Build history of the part. All positions in model axes, mm. A direction names the side the tool comes from. Round coordinates to 2 decimals unless told otherwise and drop trailing zeros. Order: outer loops, then holes, each group sorted by start corner. A loop starts at its lowest first (then second) coordinate and runs counter-clockwise, first axis right, second up. Notation, with made-up numbers: (74.5, 54.5) -> (131.5, 54.5) arc R25 cw to (131.5, 75.5) -> close; hole circle Ø6 at (69.25, -17.75). An arc over 180 degrees is marked (long way). Use a Markdown table: item, result. Add a question column.
Item 1: Two-plate mould, pull along Y, no slides. Class faces 1 (the face through (6.794, -4.514, 1.62)), 2 (the face through (0, -6, -8)), 3 (the face through (0.48, -0.25, 14.84)): released by +Y, released by -Y, zero draft, split by the parting line, or undercut.
Item 2: Slice it at A-A, the plane z = 11. Give the cut face in (x, y), plus the area to 3 significant figures.
Item 3: Pin check, flat tips, straight feed: pin 1 (4 mm diameter, centred on x = 3, z = 3.5, fed in from +Y); pin 2 (2 mm diameter, centred on x = 6, z = 7, fed in from -Y); pin 3 (8 mm diameter, centred on y = -1.5, z = -10, fed in from +X). Stop position of each tip, or through.
Item 4: Probe L1, parallel to Z at x = -6, y = -3.25; L2, parallel to Z at x = -2.75, y = -4.75 (3 decimals); L3, parallel to Y at x = 6.5, z = 13.5. List the from-to ranges inside material, lowest first.
Item 5: Slice it at B-B, the plane z = -12. Give the cut face in (x, y).
Item 6: 3-axis set-ups, long thin cutter, end or side, ignore diameter. For faces 4 (the face through (0, -10, 5)), 5 (the face through (-1.6, -5, 0.9)), 6 (the face through (-6.2, -0.1, 1.5)): which of +Z, -Z, +X, -X, +Y, -Y reach the whole face in a straight line?
from build123d import *

# Parameters (mm, degrees)
CUT_EXTRUDE4_DEPTH = 23.891046285
FILLET1_R          = 0.4
FILLET2_R          = 0.4
FILLET3_R          = 0.3


with BuildPart() as part:
    # Sketch3 → Revolve2 (revolve)
    with BuildSketch(Plane(origin=(0, 0, 0), x_dir=(0, 0, -1), z_dir=(1, 0, 0))):
        Polygon((-16.5, 0), (-16.5, 8.004748036), (-7.5, 10), (-1.5, 10), (-1.5, 6), (16.5, 6), (16.5, 0), align=None)
    revolve(axis=Axis((0, 0, -16.5), (0, 0, 1)))

    # Sketch14 → Cut-Extrude4 (cut, through all)
    with BuildSketch(Plane(origin=(0, 0, 1.5), x_dir=(-1, 0, 0), z_dir=(0, 0, -1))):
        Polygon((-9.531762002, 0), (-4.326626661, -9.01555887), (0.878508679, -18.03111774), (-12.531762002, -18.03111774), (-12.531762002, 18.03111774), (0.878508679, 18.03111774), (-4.326626661, 9.01555887), align=None)
    cut_extrude4 = extrude(amount=-CUT_EXTRUDE4_DEPTH, mode=Mode.SUBTRACT)

    # Mirror1: Cut-Extrude4 across plane
    add(cut_extrude4.mirror(Plane(origin=(0, 0, 0), x_dir=(0, 0, 1), z_dir=(1, 0, 0))), mode=Mode.SUBTRACT)

    # Sketch16 → Cut-Revolve1 (revolve, cut)
    with BuildSketch(Plane(origin=(0, 0, 0), x_dir=(0, 0, -1), z_dir=(1, 0, 0)), mode=Mode.PRIVATE) as cut_revolve1_sk:
        with BuildLine():
            Line((-1.5, 6), (-1.716506351, 5.625))
            ThreePointArc((-1.716506351, 5.625), (-1.716506351, 5.375), (-1.5, 5.25))
            Line((-1.5, 5.25), (-0.225098536, 5.25))
            ThreePointArc((-0.225098536, 5.25), (0.035373731, 5.27278837), (0.287931679, 5.340461069))
            Line((0.287931679, 5.340461069), (2.1, 6))
            Line((2.1, 6), (-1.5, 6))
        make_face()
        Polygon((13.8, 6), (16.5, 4.441154273), (16.5, 6), align=None)
    revolve(cut_revolve1_sk.sketch.rotate(Axis((0, 0, 16.5), (0, 0, -1)), 180), axis=Axis((0, 0, 16.5), (0, 0, -1)), mode=Mode.SUBTRACT)

    # Cut-Extrude2 cone 1 section (through the dimple's axis) → Cut-Extrude2 (revolve, cut)
    with BuildSketch(Plane(origin=(0, 0, 16.5), x_dir=(0, -1, 0), z_dir=(1, 0, 0))):
        Polygon((0, 0), (1.5, 0), (0, 2.598076211), align=None)
    revolve(axis=Axis((0, 0, 16.5), (0, 0, -1)), mode=Mode.SUBTRACT)

    # Cut-Extrude5 cone 1 section (through the dimple's axis) → Cut-Extrude5 (revolve, cut)
    with BuildSketch(Plane(origin=(0, 0, -16.5), x_dir=(0, 1, 0), z_dir=(1, 0, 0))):
        Polygon((0, 0), (1.5, 0), (0, 2.598076211), align=None)
    revolve(axis=Axis((0, 0, -16.5), (0, 0, 1)), mode=Mode.SUBTRACT)

    # Fillet1
    fillet1_edges = [part.edges().sort_by_distance(p)[0] for p in [
        (0, -8.004748036, 16.5),
    ]]
    fillet(fillet1_edges, radius=FILLET1_R)

    # Fillet2
    fillet2_edges = [part.edges().sort_by_distance(p)[0] for p in [
        (0, -10, 1.5),
        (6.929194331, -4.507779435, 1.5),
        (6.929194331, 4.507779435, 1.5),
        (0, 10, 1.5),
        (-6.929194331, -4.507779435, 1.5),
        (-6.929194331, 4.507779435, 1.5),
    ]]
    fillet(fillet2_edges, radius=FILLET2_R)

    # Fillet3
    fillet3_edges = [part.edges().sort_by_distance(p)[0] for p in [
        (0, 1.5, 16.5),
        (0, -1.5, -16.5),
    ]]
    fillet(fillet3_edges, radius=FILLET3_R)


solid = part.part
Check sheet entries:
| question | item | result |
|---|---|---|
| 1 | face 1 | released by -Y |
| 1 | face 2 | split by the parting line |
| 1 | face 3 | undercut |
| 2 | outline | (-9.21, -0.56) -> (-5.09, -7.69) arc R9.22 ccw to (5.09, -7.69) -> (9.21, -0.56) arc R9.22 ccw to (9.21, 0.56) -> (5.09, 7.69) arc R9.22 ccw to (-5.09, 7.69) -> (-9.21, 0.56) arc R9.22 ccw to start |
| 2 | area | 246 mm2 |
| 3 | pin 1 | y = 9.95 |
| 3 | pin 2 | y = -7.85 |
| 3 | pin 3 | x = 6 |
| 4 | L1 | 1.5 to 16.5 |
| 4 | L2 | -14.686 to -0.695, 1.75 to 16.5 |
| 4 | L3 | -5.25 to 5.25 |
| 5 | outline | circle Ø12 at (0, 0) |
| 6 | face 4 | +Z, -Z, -Y |
| 6 | face 5 | none |
| 6 | face 6 | -Z |
